from build123d import *

# Parameters (mm, degrees)
F0_W          = 44.2
F0_H          = 9.6
F0_W_2        = 12
F0_H_2        = 7
F0_W_3        = 0.2
F0_H_3        = 8.6
F1_DEPTH      = 2.4
F2_R          = 0.5
F3_W          = 44.2
F3_H          = 1.2
F4_DEPTH      = 1.6
F5_W          = 44.2
F5_H          = 1.2
F6_DEPTH      = 1.6
F8_DEPTH      = 1.6
F10_DEPTH     = 1.6
F11_R         = 0.5
F12_T1_DEPTH  = 3.7
F12_T3_DEPTH  = 3.7
F12_T6_ANGLE  = 90
F12_T8_ANGLE  = 90
F12_T10_ANGLE = 90
F12_T12_ANGLE = 90


# Not quite as in the source:
# - a fillet or chamfer that OpenCascade refuses, or shapes differently, is made with other operations: its cross-section is extruded or revolved along the edge and cut away or added
# - a feature names something its author has since deleted; it is built from what else it names


with BuildPart() as f1:
    # F0 (on Front) → F1 (new body)
    with BuildSketch(Plane.XZ):
        with Locations((58.0827572465, 2.8)):
            Rectangle(F0_W, F0_H)
        with Locations((43.2827572465, 2.8)):
            Rectangle(F0_W_2, F0_H_2, mode=Mode.SUBTRACT)
        with Locations((50.6827572465, 2.8)):
            Rectangle(F0_W_3, F0_H_3, mode=Mode.SUBTRACT)
        with Locations((58.0827572465, 2.8)):
            Rectangle(F0_W_2, F0_H_2, mode=Mode.SUBTRACT)
        with Locations((65.4827572465, 2.8)):
            Rectangle(F0_W_3, F0_H_3, mode=Mode.SUBTRACT)
        with Locations((72.8827572465, 2.8)):
            Rectangle(F0_W_2, F0_H_2, mode=Mode.SUBTRACT)
    extrude(amount=F1_DEPTH)

    # F2
    f2_edges = [f1.edges().sort_by_distance(p)[0] for p in [
        (43.282757, -2.4, 6.3),
        (37.282757, -2.4, 2.8),
        (49.282757, -2.4, 2.8),
        (58.082757, -2.4, 6.3),
        (52.082757, -2.4, 2.8),
        (58.082757, -2.4, -0.7),
        (43.282757, -2.4, -0.7),
        (64.082757, -2.4, 2.8),
        (66.882757, -2.4, 2.8),
        (72.882757, -2.4, -0.7),
        (72.882757, -2.4, 6.3),
        (78.882757, -2.4, 2.8),
    ]]
    fillet(f2_edges, radius=F2_R)

    # F3 (on face) → F4 (join)
    with BuildSketch(Plane(origin=(0, 0, -2), x_dir=(1, 0, 0), z_dir=(0, 0, -1))):
        with Locations((58.0827572465, 1.8)):
            Rectangle(F3_W, F3_H)
    extrude(amount=F4_DEPTH)

    # F5 (on face) → F6 (join)
    with BuildSketch(Plane.XY.offset(7.6)):
        with Locations((58.0827572465, -1.8)):
            Rectangle(F5_W, F5_H)
    extrude(amount=F6_DEPTH)

    # F7 (on face) → F8 (join)
    with BuildSketch(Plane(origin=(35.9827572465, 0, 0), x_dir=(0, -1, 0), z_dir=(-1, 0, 0))):
        Polygon((2.4, -3.6), (2.4, 9.2), (1.2, 9.2), (1.2, 7.6), (1.2, -2), (1.2, -3.6), align=None)
    extrude(amount=F8_DEPTH)

    # F9 (on face) → F10 (join)
    with BuildSketch(Plane.YZ.offset(80.1827572465)):
        Polygon((-1.2, 9.2), (-2.4, 9.2), (-2.4, -3.6), (-1.2, -3.6), (-1.2, -2), (-1.2, 7.6), align=None)
    extrude(amount=F10_DEPTH)

    # F11
    f11_edges = [f1.edges().sort_by_distance(p)[0] for p in [
        (58.082757, -2.4, 9.2),
        (81.782757, -2.4, 2.8),
        (58.082757, -2.4, -3.6),
        (34.382757, -2.4, 2.8),
    ]]
    fillet(f11_edges, radius=F11_R)

    # F12: fillet of radius 1 on 8 edges, made by hand

    # F12_s2 → F12_t1 (cut)
    with BuildSketch(Plane.XZ.offset(-2.5)):
        with BuildLine():
            ThreePointArc((36.9827572465, 7.6), (36.2756504653, 7.3071067812), (35.9827572465, 6.6))
            Line((35.9827572465, 6.6), (35.9827572465, 7.6))
            Line((35.9827572465, 7.6), (36.9827572465, 7.6))
        make_face()
        with BuildLine():
            ThreePointArc((35.9827572465, -1), (36.2756504653, -1.7071067812), (36.9827572465, -2))
            Line((36.9827572465, -2), (35.9827572465, -2))
            Line((35.9827572465, -2), (35.9827572465, -1))
        make_face()
        with BuildLine():
            ThreePointArc((80.1827572465, -1), (79.8898640277, -1.7071067812), (79.1827572465, -2))
            Line((79.1827572465, -2), (80.1827572465, -2))
            Line((80.1827572465, -2), (80.1827572465, -1))
        make_face()
        with BuildLine():
            ThreePointArc((80.1827572465, 6.6), (79.8898640277, 7.3071067812), (79.1827572465, 7.6))
            Line((79.1827572465, 7.6), (80.1827572465, 7.6))
            Line((80.1827572465, 7.6), (80.1827572465, 6.6))
        make_face()
    extrude(amount=F12_T1_DEPTH, mode=Mode.SUBTRACT)

    # F12_s4 → F12_t3 (cut)
    with BuildSketch(Plane.XZ.offset(-1.3)):
        with BuildLine():
            ThreePointArc((80.7827572465, 9.2), (81.4898640277, 8.9071067812), (81.7827572465, 8.2))
            Line((81.7827572465, 8.2), (81.7827572465, 9.2))
            Line((81.7827572465, 9.2), (80.7827572465, 9.2))
        make_face()
        with BuildLine():
            ThreePointArc((81.7827572465, -2.6), (81.4898640277, -3.3071067812), (80.7827572465, -3.6))
            Line((80.7827572465, -3.6), (81.7827572465, -3.6))
            Line((81.7827572465, -3.6), (81.7827572465, -2.6))
        make_face()
        with BuildLine():
            ThreePointArc((34.3827572465, -2.6), (34.6756504653, -3.3071067812), (35.3827572465, -3.6))
            Line((35.3827572465, -3.6), (34.3827572465, -3.6))
            Line((34.3827572465, -3.6), (34.3827572465, -2.6))
        make_face()
        with BuildLine():
            ThreePointArc((35.3827572465, 9.2), (34.6756504653, 8.9071067812), (34.3827572465, 8.2))
            Line((34.3827572465, 8.2), (34.3827572465, 9.2))
            Line((34.3827572465, 9.2), (35.3827572465, 9.2))
        make_face()
    extrude(amount=F12_T3_DEPTH, mode=Mode.SUBTRACT)

    # F12_s5 → F12_t6 (revolve, cut)
    with BuildSketch(Plane.YZ.offset(35.3827572465)):
        with BuildLine():
            ThreePointArc((-2.4, 8.7), (-2.2535533906, 9.0535533906), (-1.9, 9.2))
            Line((-1.9, 9.2), (-2.4, 9.2))
            Line((-2.4, 9.2), (-2.4, 8.7))
        make_face()
    revolve(axis=Axis((35.3827572465, -2.4, 8.2), (0, -1, 0)), revolution_arc=F12_T6_ANGLE, mode=Mode.SUBTRACT)

    # F12_s7 → F12_t8 (revolve, cut)
    with BuildSketch(Plane.XY.offset(-2.6)):
        with BuildLine():
            ThreePointArc((34.8827572465, -2.4), (34.5292038559, -2.2535533906), (34.3827572465, -1.9))
            Line((34.3827572465, -1.9), (34.3827572465, -2.4))
            Line((34.3827572465, -2.4), (34.8827572465, -2.4))
        make_face()
    revolve(axis=Axis((35.3827572465, -2.4, -2.6), (0, -1, 0)), revolution_arc=F12_T8_ANGLE, mode=Mode.SUBTRACT)

    # F12_s9 → F12_t10 (revolve, cut)
    with BuildSketch(Plane.YZ.offset(80.7827572465)):
        with BuildLine():
            ThreePointArc((-2.4, -3.1), (-2.2535533906, -3.4535533906), (-1.9, -3.6))
            Line((-1.9, -3.6), (-2.4, -3.6))
            Line((-2.4, -3.6), (-2.4, -3.1))
        make_face()
    revolve(axis=Axis((80.7827572465, -2.4, -2.6), (0, -1, 0)), revolution_arc=F12_T10_ANGLE, mode=Mode.SUBTRACT)

    # F12_s11 → F12_t12 (revolve, cut)
    with BuildSketch(Plane.XY.offset(8.2)):
        with BuildLine():
            ThreePointArc((81.2827572465, -2.4), (81.6363106371, -2.2535533906), (81.7827572465, -1.9))
            Line((81.7827572465, -1.9), (81.7827572465, -2.4))
            Line((81.7827572465, -2.4), (81.2827572465, -2.4))
        make_face()
    revolve(axis=Axis((80.7827572465, -2.4, 8.2), (0, -1, 0)), revolution_arc=F12_T12_ANGLE, mode=Mode.SUBTRACT)


solid = f1.part
Verification items for the finished model (mm, model axes). A direction names the side the tool comes from. Coordinates: 2 decimals unless noted, no trailing zeros. Order: outer loops, then holes, each group sorted by start corner. A loop starts at its lowest first (then second) coordinate and runs counter-clockwise, first axis right, second up.
Item 1: Access from +Z, -Z, +X, -X, +Y, -Y to the whole of each face (thin tool, end or side, straight path). Record for faces 1 (the face through (36.28, -0.59, 7.31)), 2 (the face through (58, -2.4, 7)), 3 (the face through (79.898, -0.592, 7.299)), 4 (the face through (50.583, -1, 3)).
Filled in:
face 1: +Z, -X, +Y
face 2: +Z, -Z, +X, -X, -Y
face 3: +Z, +X, +Y
face 4: +Y, -Y
Item 2: Section check C-C, the plane z = 4. Give the number of separate pieces and of enclosed holes in the cut face, then the cut area to 3 significant figures.
Filled in:
separate pieces: 6
enclosed holes: 0
area: 22.1 mm2
Item 3: Section check B-B, the plane y = -0.45. Enter the section's corners in (x, z), then the cut area to 3 significant figures.
Filled in:
outline: (35.98, -1) arc R1 ccw to (36.98, -2) - (79.18, -2) arc R1 ccw to (80.18, -1) - (80.18, 6.6) arc R1 ccw to (79.18, 7.6) - (36.98, 7.6) arc R1 ccw to (35.98, 6.6) - close; hole (37.28, -0.7) - (49.28, -0.7) - (49.28, 6.3) - (37.28, 6.3) - close; hole (50.58, -1.5) - (50.78, -1.5) - (50.78, 7.1) - (50.58, 7.1) - close; hole (52.08, -0.7) - (64.08, -0.7) - (64.08, 6.3) - (52.08, 6.3) - close; hole (65.38, -1.5) - (65.58, -1.5) - (65.58, 7.1) - (65.38, 7.1) - close; hole (66.88, -0.7) - (78.88, -0.7) - (78.88, 6.3) - (66.88, 6.3) - close
area: 168 mm2
Item 4: Release check for a two-part mould opening along X. For faces 5 (the face through (58, -1, -2)), 6 (the face through (52.083, -1, 3)), 7 (the face through (80.183, -1, 3)) record: +X half, -X half, draft (parallel to the pull), parting line (faces both ways), or undercut.
Filled in:
face 5: draft
face 6: undercut
face 7: +X half
Item 5: Depth check by flat-ended pin: pin 1 (1 mm diameter, centred on x = 74, y = -0.5, fed in from -Z). Enter the tip coordinate at first touch or a pass-through.
Filled in:
pin 1: stops at z = -2
Item 6: Section check A-A, the plane x = 68.5. Enter the section's corners in (y, z), then the cut area to 3 significant figures.
Filled in:
outline: (-2.4, -3.1) arc R0.5 ccw to (-1.9, -3.6) - (-1.2, -3.6) - (-1.2, -2) - (0, -2) - (0, -0.7) - (-1.9, -0.7) arc R0.5 ccw to (-2.4, -1.2) - close; (-2.4, 6.8) arc R0.5 ccw to (-1.9, 6.3) - (0, 6.3) - (0, 7.6) - (-1.2, 7.6) - (-1.2, 9.2) - (-1.9, 9.2) arc R0.5 ccw to (-2.4, 8.7) - close
area: 9.87 mm2
Item 7: Material ranges on L1, parallel to X at y = -0.55, z = 0; L2, parallel to X at y = -0.95, z = -0.75; L3, parallel to Z at x = 42, y = -0.25, recorded low to high.
Filled in:
L1: x = 35.98 to 37.28, 49.28 to 50.58, 50.78 to 52.08, 64.08 to 65.38, 65.58 to 66.88, 78.88 to 80.18
L2: x = 35.98 to 50.58, 50.78 to 65.38, 65.58 to 80.18
L3: z = -2 to -0.7, 6.3 to 7.6
